Geometry: final body of the model. Coordinates: model frame, mm. Face numbers are marked on the shaded views. A direction names the side the tool comes from. Give positions to 0.01 mm unless a question says otherwise; leave off trailing zeros. Write each loop counter-clockwise with the first axis right and the second up, starting at its lowest first coordinate (ties: lowest second). Pieces come first, ordered by that corner, then holes.
Q1. Mould query, pull axis X, two halves, no side actions, for the marked faces 6, 7, 8 and 9. Classes: +X half, -X half, draft (parallel to the pull), parting line (faces both ways), or undercut.
Q2. Section C-C (x = -16.5). Return the cut outline in (y, z).
Q3. Line query: line 1 (Y direction, x = -28, z = 0); line 2 (Y direction, x = -27, z = 0); line 3 (Y direction, x = -3, z = 0). Output: solid intervals per line, ascending.
Q4. Reachability of the marked faces 1, 2, 3, 4 and 5 from +Z, -Z, +X, -X, +Y, -Y: full face, straight path, thin tool, end or side. Return the list, or none.
Q5. Pin query (flat end, axial travel): pin 1 Ø12 at (x, y) = (-9, 20) entering from +Z; pin 2 Ø3 at (x, z) = (-9, -13.5) entering from -Y; pin 3 Ø1.5 at (x, z) = (-17, -11) entering from -Y. Return the tip coordinate at first contact, or that it passes through.
Q6. Section D-D (z = 14). Return the cut outline in (x, y), plus the area to 3 significant figures.
from build123d import *

# Parameters (mm, degrees)
FILLET1_R = 1


with BuildPart() as part:
    # Sketch1 → Revolve1 (revolve)
    with BuildSketch(Plane.XY, mode=Mode.PRIVATE) as revolve1_sk:
        Polygon((0, 10), (0, 25), (-2.5, 25), (-2.5, 20), (-27.5, 20), (-27.5, 25), (-30, 25), (-30, 17.5), (-25, 17.5), (-25, 7.5), (-30, 7.5), (-30, 5), (5, 5), (5, 10), align=None)
    revolve(revolve1_sk.sketch.rotate(Axis((0, 0, 0), (-1, 0, 0)), 90), axis=Axis((0, 0, 0), (-1, 0, 0)))

    # Fillet1
    fillet1_edges = [part.edges().sort_by_distance(p)[0] for p in [
        (-30, 0, 7.5),
    ]]
    fillet(fillet1_edges, radius=FILLET1_R)


solid = part.part
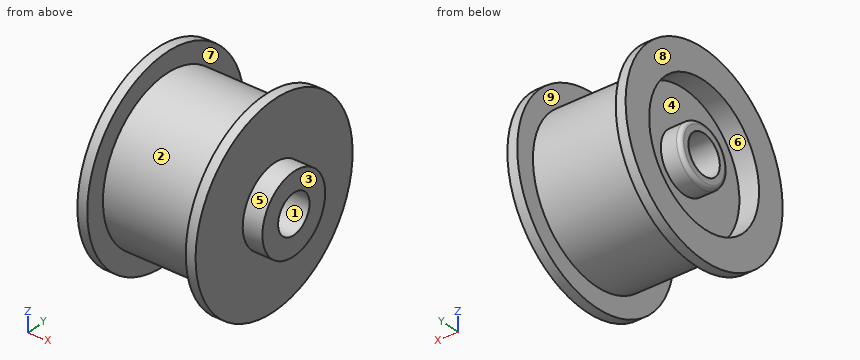
Computed:
1. face 6: draft
1. face 7: undercut
1. face 8: -X half
1. face 9: undercut
2. outline: circle Ø40 at (0, 0); hole circle Ø10 at (0, 0)
3. line 1: y = -25 to -17.5, -7.5 to -5, 5 to 7.5, 17.5 to 25
3. line 2: y = -20 to -17.5, -7.5 to -5, 5 to 7.5, 17.5 to 20
3. line 3: y = -20 to -5, 5 to 20
4. face 1: +X, -X
4. face 2: none
4. face 3: +Z, -Z, +X, +Y, -Y
4. face 4: -X
4. face 5: +X
5. pin 1: stops at z = 14.28
5. pin 2: stops at y = -16
5. pin 3: stops at y = -17.17
6. outline: (-30, -20.71) - (-27.5, -20.71) - (-27.5, -14.28) - (-2.5, -14.28) - (-2.5, -20.71) - (0, -20.71) - (0, 20.71) - (-2.5, 20.71) - (-2.5, 14.28) - (-27.5, 14.28) - (-27.5, 20.71) - (-30, 20.71) - (-30, 10.5) - (-25, 10.5) - (-25, -10.5) - (-30, -10.5) - close
6. area: 816 mm2
